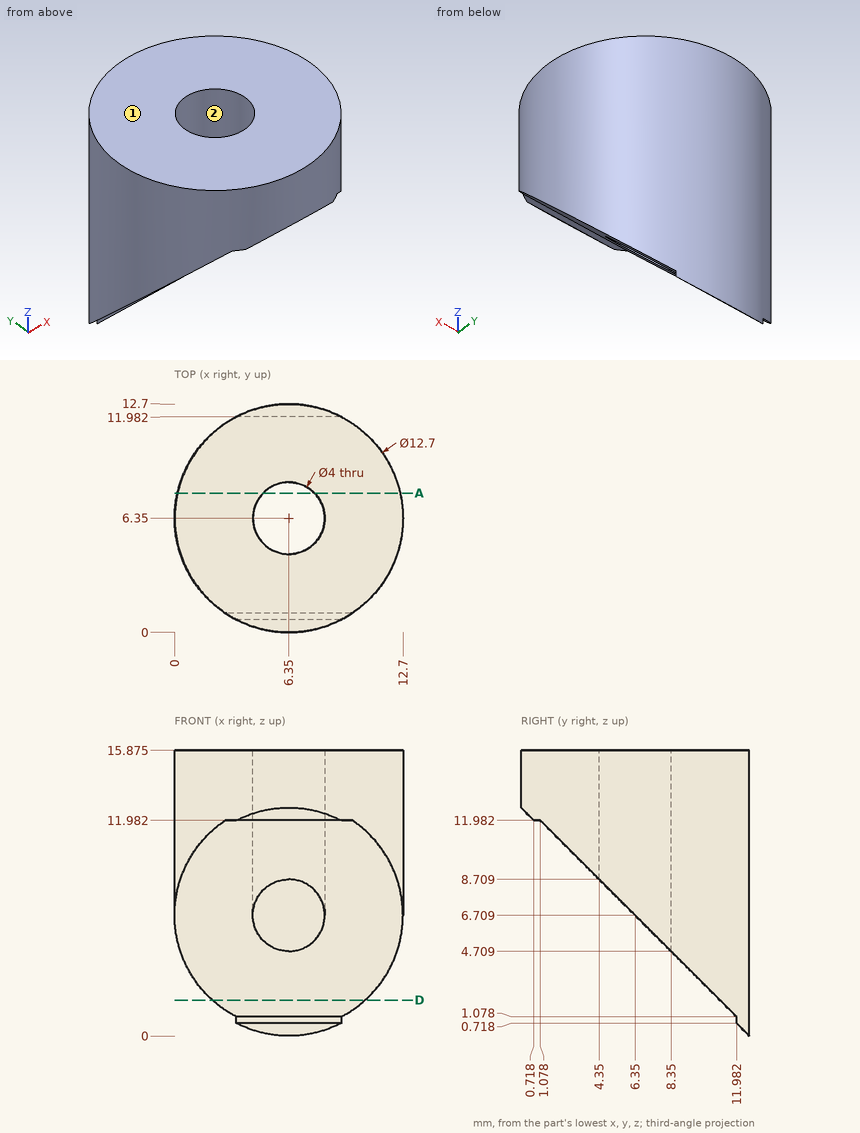
Here's the drawing with two shaded views (mm, measured from the low corner). I have some questions. Round coordinates to 2 decimals unless told otherwise and drop trailing zeros. Loops run counter-clockwise (first coordinate to the right, second up) from the corner with the lowest first, then second, coordinate; pieces in that order, holes last. Notation, with made-up numbers: M 85,-14 L 119,-14 A21 ccw 119,0 Z; hole C 88.5,81 d1. An arc over 180 degrees is marked long. Put each result on its own line as item: value.
Q1. I need wall thicknesses on probe 1 along X at (y, z) = (6.35, 8.5); probe 2 along Y at (x, z) = (6.35, 7.75). Which ranges of each line are inside material? Lowest first, please.
Check result:
probe 1: 0 to 4.35, 8.35 to 12.7
probe 2: 8.35 to 12.7
Q2. For pin 1 (1.5 mm diameter, centred on x = 11, z = 7.5, fed in from +Y); pin 2 (6 mm diameter, centred on y = 9.5, z = 6, fed in from -X); pin 3 (4 mm diameter, centred on x = 9.5, z = 8, fed in from -Y), each with a flat end and sliding along its axis, tell me the tip position at first contact or that it passes through.
Check result:
pin 1: y = 11.36
pin 2: x = 0
pin 3: y = 3.06
Q3. Imagine slicing it at D-D (z = 2). Write out the boundary of the cut face in (x, y).
Check result:
outline: M 2.09,11.06 L 10.61,11.06 A6.35 ccw Z
Q4. Imagine slicing it at A-A (y = 7.75). Write out the boundary of the cut face in (x, z) (1 decimal).
Check result:
outline: M 0.2,5.3 L 4.9,5.3 L 4.9,15.9 L 0.2,15.9 Z; M 7.8,5.3 L 12.5,5.3 L 12.5,15.9 L 7.8,15.9 Z
Q5. Thinking about a two-plate mould opening in Z: for the marked faces 1 and 2, which applies, released by +Z, released by -Z, zero draft, split by the parting line, or undercut?
Check result:
face 1: released by +Z
face 2: zero draft
